Job drawing, mm, ordinate dimensions from the low corner. One solid piece. A direction names the side the tool comes from. Round coordinates to 2 decimals unless told otherwise and drop trailing zeros. Loops run counter-clockwise (first coordinate to the right, second up) from the corner with the lowest first, then second, coordinate; pieces in that order, holes last.
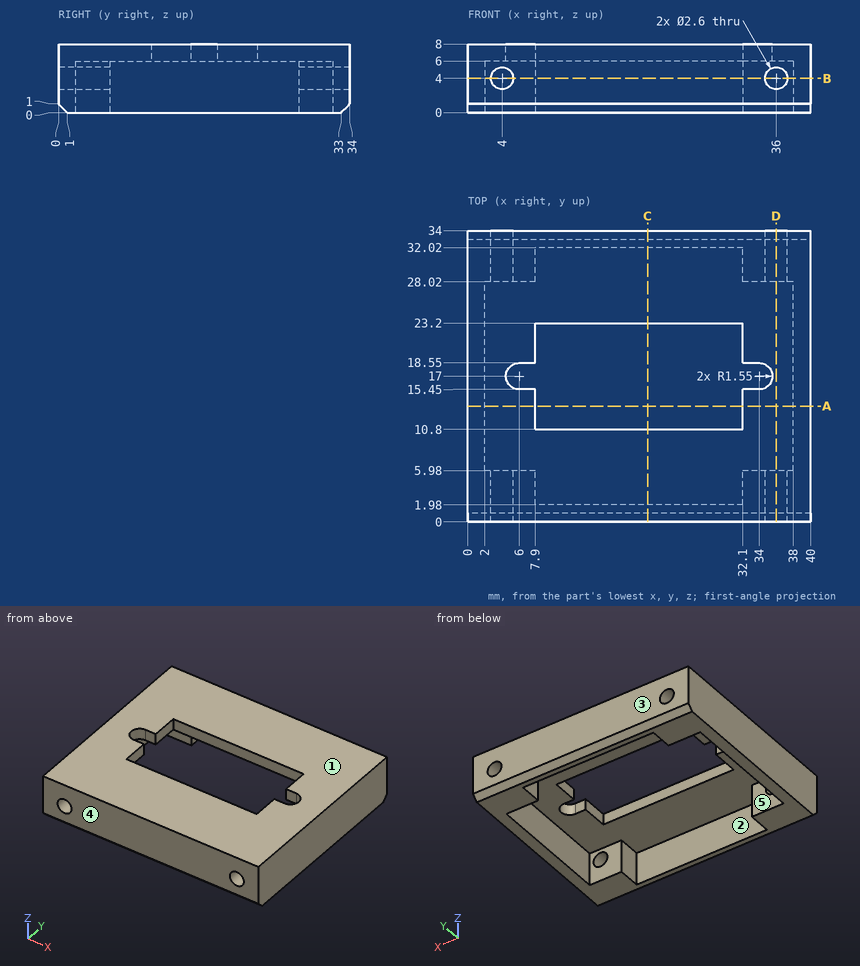
(1) Pin check, flat tip, straight feed: P1, Ø10, axis at x = 26, y = 10.5, coming from the -Z side. Stop position of the tip, or through.
Responses:
P1: stops at z = 6
(2) Slice it at D-D on x = 36. List the corners of the cut face in (y, z).
Responses:
outline: (0, 1) - (1, 0) - (5.98, 0) - (5.98, 2.7) - (0, 2.7) - close; (0, 5.3) - (5.98, 5.3) - (5.98, 6) - (28.02, 6) - (28.02, 5.3) - (34, 5.3) - (34, 8) - (0, 8) - close; (28.02, 0) - (33, 0) - (34, 1) - (34, 2.7) - (28.02, 2.7) - close
(3) Slice it at C-C on x = 21. List the corners of the cut face in (y, z), plus the area to 3 significant figures.
Responses:
outline: (0, 1) - (1, 0) - (1.98, 0) - (1.98, 6) - (10.8, 6) - (10.8, 8) - (0, 8) - close; (23.2, 6) - (32.02, 6) - (32.02, 0) - (33, 0) - (34, 1) - (34, 8) - (23.2, 8) - close
area: 66.0 mm2
(4) Slice it at A-A on y = 13.5. List the corners of the cut face in (x, z).
Responses:
outline: (0, 0) - (2, 0) - (2, 6) - (7.9, 6) - (7.9, 8) - (0, 8) - close; (32.1, 6) - (38, 6) - (38, 0) - (40, 0) - (40, 8) - (32.1, 8) - close
(5) Which spindle directions (+Z, -Z, +X, -X, +Y, -Y) get a long thin tool onto all of the face, cutting with end or side? Do the marked faces 1 and 2. Say none if no direction does.
Responses:
face 1: +Z, +X, -X, +Y, -Y
face 2: -Z
(6) Pull direction Y, two halves, no side cores. Call the marked faces 3, 4 and 5: +Y half, -Y half, draft (parallel to the pull), parting line (faces both ways), or undercut.
Responses:
face 3: +Y half
face 4: -Y half
face 5: undercut
(7) Slice it at B-B on z = 4. Count the separate pieces of the cut face and the enclosed holes in it, plus the area to 3 significant figures.
Responses:
separate pieces: 4
enclosed holes: 0
area: 311 mm2
(8) Probe line 1 (X direction, y = 2.65, z = 4); line 2 (Y direction, x = 25, z = 3.5); line 3 (X direction, y = 7.5, z = 5.25). List the from-to ranges inside material, lowest first.
Responses:
line 1: x = 0 to 2.7, 5.3 to 7.9, 32.1 to 34.7, 37.3 to 40
line 2: y = 0 to 1.98, 32.02 to 34
line 3: x = 0 to 2, 38 to 40
